The model under review builds one solid part; all positions refer to its coordinate system, in mm. Give positions to 0.01 mm unless a question says otherwise; leave off trailing zeros. Order: outer loops, then holes, each group sorted by start corner. A loop starts at its lowest first (then second) coordinate and runs counter-clockwise, first axis right, second up. Notation, with made-up numbers: (67.5, 33.5) - (85.5, 33.5) arc R12 ccw to (85.5, 45.5) - close; hole circle Ø11 at (-10.75, 67.25). An arc over 180 degrees is marked (long way). Use CSV: the item, a comma, the result in double quotes. Start each with the question number.
1. For pin 1 (2 mm diameter, centred on x = 9, z = 5, fed in from +Y); pin 2 (1 mm diameter, centred on x = -7, z = -0.5, fed in from +Y); pin 3 (2 mm diameter, centred on y = 10.5, z = 2.5, fed in from +X), all flat-tipped, find the tip position at first contact; note any pin that passes through.
2. Take a section at A-A, the plane z = 3.5. State the section outline as (x, y) points, then the cut area to 3 significant figures.
3. To check wall thickness, follow line 1 (X direction, y = -16, z = -0.75); line 2 (Y direction, x = 24, z = 6); line 3 (Y direction, x = 0, z = 5.5). State the ranges of each line that lie inside material, in increasing order. Write a range as [from, to].
4. Take a section at B-B, the plane y = 0. State the section outline as (x, z) points.
```python
from build123d import *

# Parameters (mm, degrees)
SKETCH_1_R          = 25
EXTRUDE_1_DEPTH     = 7
SKETCH_2_R          = 20
CUT_EXTRUDE_1_DEPTH = 31
SCALE_1_SCALE       = 1.5


with BuildPart() as part:
    # 草图1 → 凸台-拉伸1 (new body)
    with BuildSketch(Plane.XY):
        Circle(SKETCH_1_R)
    extrude(amount=EXTRUDE_1_DEPTH)

    # 草图2 → 切除-拉伸1 (cut)
    with BuildSketch(Plane.XY.offset(7)):
        Circle(SKETCH_2_R)
    extrude(amount=-CUT_EXTRUDE_1_DEPTH, mode=Mode.SUBTRACT)

    # 草图7 → 切除-旋转1 (revolve, cut)
    with BuildSketch(Plane(origin=(0, 0, 0), x_dir=(0, -1, 0), z_dir=(-1, 0, 0)), mode=Mode.PRIVATE) as cut_revolve_1_sk:
        with BuildLine():
            Line((-20, 7), (-25, 7))
            Line((-25, 7), (-25, 0))
            Line((-25, 0), (-20, 0))
            ThreePointArc((-20, 0), (-23.5, 3.5), (-20, 7))
        make_face()
    revolve(cut_revolve_1_sk.sketch.rotate(Axis((0, 0, 0), (0, 0, 1)), 90), axis=Axis((0, 0, 0), (0, 0, 1)), mode=Mode.SUBTRACT)


with BuildPart() as part_1:
    # 缩放比例1: scaled about (0, 0, 3.5)
    add(part.part.scale(SCALE_1_SCALE).moved(Location((0, 0, -1.75))))


solid = part_1.part
```
Determined:
1,pin 1,"stops at y = 34.2"
1,pin 2,"stops at y = 33.19"
1,pin 3,"stops at x = 33.89"
2,outline,"circle Ø70.5 at (0, 0); hole circle Ø60 at (0, 0)"
2,area,"1,080 mm²"
3,line 1,"x = [-28.96, -25.38], [25.38, 28.96]"
3,line 2,"y = [-24.95, -18], [18, 24.95]"
3,line 3,"y = [-34.85, -30], [30, 34.85]"
4,outline,"(-30, -1.75) - (-30, 8.75) arc R5.25 ccw to start; (30, -1.75) arc R5.25 ccw to (30, 8.75) - close"
